from build123d import *

# Parameters (mm, degrees)
BOSS_EXTRUDE1_DEPTH     = 10.8
BOSS_EXTRUDE2_DEPTH     = 10.64
CUT_EXTRUDE1_DEPTH      = 39.168054705
CUT_EXTRUDE1_DEPTH_BACK = 39.168054705
SKETCH5_R               = 5
FILLET1_R               = 1
SKETCH6_W               = 21.28
SKETCH6_H               = 16.18
BOSS_EXTRUDE3_DEPTH     = 12
SKETCH7_W               = 5
SKETCH7_H               = 21.281328743
BOSS_EXTRUDE4_DEPTH     = 56.83
SKETCH8_W               = 21.284331222
SKETCH8_H               = 16.18
BOSS_EXTRUDE5_DEPTH     = 7.19
FILLET3_R               = 3
SKETCH9_R               = 2.2
CUT_EXTRUDE2_DEPTH      = 85.918196519
SKETCH10_R              = 2
CUT_EXTRUDE3_DEPTH      = 85.918196519
SKETCH11_W              = 24.977296572
SKETCH11_H              = 9.721484234
CUT_EXTRUDE4_DEPTH      = 71.220021919
CUT_EXTRUDE5_REACH      = 86.898


with BuildPart() as part:
    # Sketch2 → Boss-Extrude1 (new body)
    with BuildSketch(Plane.XY):
        Polygon((-10.1, 0), (0, 0), (0, 7), (-6.25480432, 7), (-10.1, 1.709943763), align=None)
        Polygon((0, 0), (10.1, 0), (10.1, 1.709943763), (6.25480432, 7), (0, 7), align=None)
    extrude(amount=BOSS_EXTRUDE1_DEPTH)

    # Sketch4 → Boss-Extrude2 (add, symmetric)
    with BuildSketch(Plane.XY):
        Polygon((-3.8, 0), (-3.8, -4.8), (-30, -4.8), (-30, -20.98), (30, -20.98), (30, -4.8), (3.8, -4.8), (3.8, 0), align=None)
    extrude(amount=BOSS_EXTRUDE2_DEPTH, both=True)

    # Sketch5 → Cut-Extrude1 (cut, two sides: drawn at the far end of the back side and taken through both)
    with BuildSketch(Plane.XY.offset(-CUT_EXTRUDE1_DEPTH_BACK)):
        with Locations((-22.790976064, -22.227391232)):
            Circle(SKETCH5_R)
        with Locations((22.790976064, -22.227391232)):
            Circle(SKETCH5_R)
    extrude(amount=CUT_EXTRUDE1_DEPTH + CUT_EXTRUDE1_DEPTH_BACK, mode=Mode.SUBTRACT)

    # Fillet1
    fillet1_edges = [part.edges().sort_by_distance(p)[0] for p in [
        (-10.1, 0, 5.4),
        (-10.1, 1.709943763, 5.4),
        (-6.25480432, 7, 5.4),
        (6.25480432, 7, 5.4),
        (10.1, 1.709943763, 5.4),
        (10.1, 0, 5.4),
    ]]
    fillet(fillet1_edges, radius=FILLET1_R)

    # Sketch6 → Boss-Extrude3 (add)
    with BuildSketch(Plane(origin=(30, 0, 0), x_dir=(0, 0, -1), z_dir=(1, 0, 0))):
        with Locations((0, -12.89)):
            Rectangle(SKETCH6_W, SKETCH6_H)
    extrude(amount=BOSS_EXTRUDE3_DEPTH)

    # Sketch7 → Boss-Extrude4 (add)
    with BuildSketch(Plane(origin=(0, -4.8, 0), x_dir=(1, 0, 0), z_dir=(0, 1, 0))):
        with Locations((39.5, 0.000664372)):
            Rectangle(SKETCH7_W, SKETCH7_H)
    extrude(amount=BOSS_EXTRUDE4_DEPTH)

    # Sketch8 → Boss-Extrude5 (add)
    with BuildSketch(Plane.ZY.offset(-37)):
        with Locations((0.000836868, 43.94)):
            Rectangle(SKETCH8_W, SKETCH8_H)
    extrude(amount=BOSS_EXTRUDE5_DEPTH)

    # Fillet3
    fillet3_edges = [part.edges().sort_by_distance(p)[0] for p in [
        (42, -20.98, 0),
        (42, 52.03, -0.000664372),
    ]]
    fillet(fillet3_edges, radius=FILLET3_R)

    # Sketch9 → Cut-Extrude2 (cut, through all)
    with BuildSketch(Plane.XZ.offset(20.98)):
        with Locations((32.632878078, 0)):
            Circle(SKETCH9_R)
    extrude(amount=-CUT_EXTRUDE2_DEPTH, mode=Mode.SUBTRACT)

    # Sketch10 → Cut-Extrude3 (cut, through all)
    with BuildSketch(Plane.XZ.offset(20.98)):
        with Locations((0.000925951, 0)):
            Circle(SKETCH10_R)
    extrude(amount=-CUT_EXTRUDE3_DEPTH, mode=Mode.SUBTRACT)

    # Sketch11 → Cut-Extrude4 (cut, through all)
    with BuildSketch(Plane.XY.offset(10.8)):
        with Locations((-0.121132817, 4.060742117)):
            Rectangle(SKETCH11_W, SKETCH11_H)
    extrude(amount=-CUT_EXTRUDE4_DEPTH, mode=Mode.SUBTRACT)

    # Sketch13 → Cut-Extrude5 (cut, up to next)
    with BuildSketch(Plane.XZ.offset(20.98), mode=Mode.PRIVATE) as cut_extrude5_sk1:
        with BuildLine():
            ThreePointArc((-8.827441341, 6.170359992), (-7.827441341, 5.170359992), (-6.827441341, 6.170359992))
            ThreePointArc((-6.827441341, 6.170359992), (-7.827441341, 7.170359992), (-8.827441341, 6.170359992))
        make_face()
    cut_extrude5_tool1 = extrude(cut_extrude5_sk1.sketch, amount=-CUT_EXTRUDE5_REACH, mode=Mode.PRIVATE) & part.part
    # Sketch13 → Cut-Extrude5 (cut, up to next)
    with BuildSketch(Plane.XZ.offset(20.98), mode=Mode.PRIVATE) as cut_extrude5_sk2:
        with BuildLine():
            ThreePointArc((-13.327441341, 6.170359992), (-14.327441341, 7.170359992), (-15.327441341, 6.170359992))
            ThreePointArc((-15.327441341, 6.170359992), (-14.327441341, 5.170359992), (-13.327441341, 6.170359992))
        make_face()
    cut_extrude5_tool2 = extrude(cut_extrude5_sk2.sketch, amount=-CUT_EXTRUDE5_REACH, mode=Mode.PRIVATE) & part.part
    add(cut_extrude5_tool1.solids().sort_by_distance((-7.827441, -20.98, 6.17036))[0], mode=Mode.SUBTRACT)
    add(cut_extrude5_tool2.solids().sort_by_distance((-14.327441, -20.98, 6.17036))[0], mode=Mode.SUBTRACT)


solid = part.part
Work out the finished part from the listing and answer in its coordinate system (mm). A direction names the side the tool comes from. Coordinates: 2 decimals unless noted, no trailing zeros. Write each loop counter-clockwise with the first axis right and the second up, starting at its lowest first coordinate (ties: lowest second). Pieces come first, ordered by that corner, then holes.
1. The part is cut by section D-D, the plane z = 4.25. Write down the section's boundary in (x, y), and give its area (3 significant figures).
Results list:
outline: (-30, -20.98) - (-27.63, -20.98) arc R5 cw to (-17.95, -20.98) - (17.95, -20.98) arc R5 cw to (27.63, -20.98) - (39, -20.98) arc R3 ccw to (42, -17.98) - (42, 49.03) arc R3 ccw to (39, 52.03) - (29.81, 52.03) - (29.81, 35.85) - (37, 35.85) - (37, -4.8) - (3.8, -4.8) - (3.8, -0.8) - (-3.8, -0.8) - (-3.8, -4.8) - (-30, -4.8) - close
area: 1,540 mm2
2. For a pull along X with two mould halves and no side action, classify faces 1 (the cylindrical face through (41.1, 51.17, -0.15)), 2 (the cylindrical face through (30.435, 43.827, 0.097)), 3 (the flat face through (11, -6, 10.64)), 4 (the cylindrical face through (22.88, -17.23, -0.15)) as +X half, -X half, draft (parallel to the pull), parting line (faces both ways), or undercut.
Results list:
face 1: +X half
face 2: undercut
face 3: draft
face 4: undercut
3. Flat-ended cylindrical pins translate along their axes: pin 1 (5 mm diameter, centred on y = 12, z = 5, fed in from -X); pin 2 (4.5 mm diameter, centred on y = -2, z = 1.5, fed in from -X); pin 3 (5 mm diameter, centred on y = 43.5, z = 0, fed in from -X). Find the tip coordinate at first contact, or state that the pin passes through.
Results list:
pin 1: stops at x = 37
pin 2: stops at x = -3.8
pin 3: stops at x = 29.81
4. Consider line 1 along Y through (x, z) = (-7.5, -5.5); line 2 along X through (y, z) = (0, 1); line 3 along Y through (x, z) = (36.5, -2). Determine where each line is inside the solid, lowest interval first.
Results list:
line 1: y = -20.98 to -4.8
line 2: x = 37 to 42
line 3: y = -20.98 to -4.8, 35.85 to 52.03
5. The part is cut by section B-B, the plane z = 0. State how many separate pieces and enclosed holes the cut face has, and give its area (3 significant figures).
Results list:
separate pieces: 4
enclosed holes: 0
area: 1,320 mm2
6. For faces 5 (the flat face through (-17, -4.8, 0)), 6 (the flat face through (42, 15, 0)), 7 (the flat face through (20, -4.8, 0)), determine the directions among +Z, -Z, +X, -X, +Y, -Y from which every point of the face is accessible in a straight line to the end or side of a thin tool.
Results list:
face 5: +Z, -Z, -X, +Y
face 6: +Z, -Z, +X, +Y, -Y
face 7: +Z, -Z
7. The part is cut by section C-C, the plane x = 33.5. Write down the section's boundary in (y, z), and give its area (3 significant figures).
Results list:
outline: (-20.98, -10.64) - (-4.8, -10.64) - (-4.8, -2.02) - (-20.98, -2.02) - close; (-20.98, 2.02) - (-4.8, 2.02) - (-4.8, 10.64) - (-20.98, 10.64) - close; (35.85, -10.64) - (52.03, -10.64) - (52.03, -2.02) - (35.85, -2.02) - close; (35.85, 2.02) - (52.03, 2.02) - (52.03, 10.64) - (35.85, 10.64) - close
area: 558 mm2
